Source: CAD feature listing. Evaluate the final solid. Frame: model axes, mm. Round coordinates to 2 decimals unless told otherwise and drop trailing zeros. Loops run counter-clockwise (first coordinate to the right, second up) from the corner with the lowest first, then second, coordinate; pieces in that order, holes last.
(1) First-contact query: pin 1 Ø1.9 at (x, z) = (199, 1.5) entering from -Y. Flat tip, straight axial feed; report the tip coordinate or a pass-through.
(2) Section B-B, the plane z = 0.7. Count the separate pieces of the cut face and the enclosed holes in it, plus the area to 3 significant figures.
(3) Section A-A, the plane x = 199. Return the cut outline in (y, z).
(4) Material intervals for probe 1 along Y at (x, z) = (226, 1.05); probe 2 along Y at (x, z) = (399, 3.1), sorted ascending.
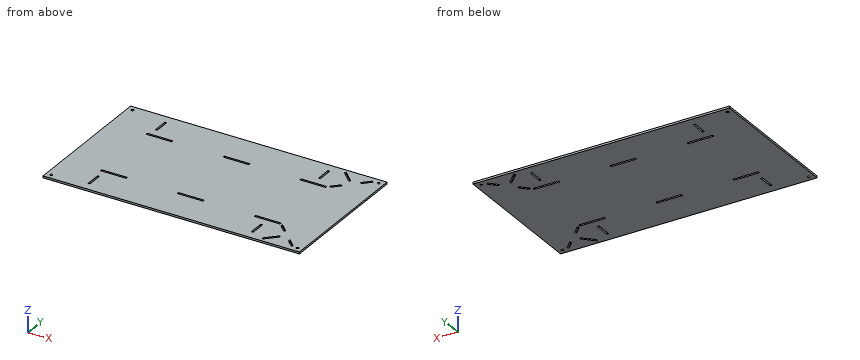
```python
from build123d import *

# Parameters (mm, degrees)
F0_W     = 3.75
F0_H     = 30
F0_W_2   = 50
F0_H_2   = 3.75
F1_DEPTH = 3.75
F3_D     = 5
F5_DEPTH = 3.75


# Not quite as in the source:
# - a feature names something its author has since deleted; it is built from what else it names


with BuildPart() as f1:
    # F0 (on Top) → F1 (new body)
    with BuildSketch(Plane.XY):
        Polygon((-37.9051826894, 0), (12.0948173106, 0), (462.0948173106, 0), (462.0948173106, 280), (62.0948173106, 280), (-37.9051826894, 280), align=None)
        with Locations((41.3065613726, 32.5)):
            Rectangle(F0_W, F0_H, mode=Mode.SUBTRACT)
        with Locations((59.4315613726, 66.875)):
            Rectangle(F0_W_2, F0_H_2, mode=Mode.SUBTRACT)
        with Locations((209.4315613726, 66.875)):
            Rectangle(F0_W_2, F0_H_2, mode=Mode.SUBTRACT)
        with Locations((359.4315613726, 32.5)):
            Rectangle(F0_W, F0_H, mode=Mode.SUBTRACT)
        with Locations((359.4315613726, 66.875)):
            Rectangle(F0_W_2, F0_H_2, mode=Mode.SUBTRACT)
        with Locations((59.4315613726, 213.125)):
            Rectangle(F0_W_2, F0_H_2, mode=Mode.SUBTRACT)
        with Locations((41.3065613726, 247.5)):
            Rectangle(F0_W, F0_H, mode=Mode.SUBTRACT)
        with Locations((209.4315613726, 213.125)):
            Rectangle(F0_W_2, F0_H_2, mode=Mode.SUBTRACT)
        with Locations((359.4315613726, 213.125)):
            Rectangle(F0_W_2, F0_H_2, mode=Mode.SUBTRACT)
        with Locations((359.4315613726, 247.5)):
            Rectangle(F0_W, F0_H, mode=Mode.SUBTRACT)
    extrude(amount=F1_DEPTH)

    # F3 (through all)
    with Locations(Plane.XY.offset(3.75)):
        with Locations((-27.9051826894, 10), (-27.9051826894, 270), (452.0948173106, 10), (452.0948173106, 270)):
            Hole(F3_D / 2)

    # F4 (on face) → F5 (cut)
    with BuildSketch(Plane.XY.offset(3.75)):
        Polygon((442.083211802, 267.3483495706), (439.4315613726, 270), (425.2894257488, 255.8578643763), (427.9410761783, 253.2062139468), align=None)
        Polygon((402.1092280247, 232.6776666521), (387.9670924009, 218.5355310284), (390.6187428304, 215.8838805989), (404.7608784541, 230.0260162227), align=None)
        Polygon((386.740880854, 273.8778619764), (384.0892304246, 271.2262115469), (405.3024338602, 250.0130081113), (407.9540842896, 252.6646585408), align=None)
        Polygon((387.9670924009, 61.4644689716), (402.1092280247, 47.3223333479), (404.7608784541, 49.9739837773), (390.6187428304, 64.1161194011), align=None)
        Polygon((405.3024338602, 29.9869918887), (384.0892304246, 8.7737884531), (386.740880854, 6.1221380236), (407.9540842896, 27.3353414592), align=None)
        Polygon((427.9410761783, 26.7937860532), (425.2894257488, 24.1421356237), (439.4315613726, 10), (442.083211802, 12.6516504294), align=None)
    extrude(amount=-F5_DEPTH, mode=Mode.SUBTRACT)


solid = f1.part
```
Output values:
1. pin 1: stops at y = 0
2. separate pieces: 1
2. enclosed holes: 20
2. area: 138,000 mm2
3. outline: (0, 0) - (65, 0) - (65, 3.75) - (0, 3.75) - close; (68.75, 0) - (211.25, 0) - (211.25, 3.75) - (68.75, 3.75) - close; (215, 0) - (280, 0) - (280, 3.75) - (215, 3.75) - close
4. probe 1: y = 0 to 65, 68.75 to 211.25, 215 to 280
4. probe 2: y = 0 to 18.38, 23.68 to 50.43, 55.73 to 224.27, 229.57 to 256.32, 261.62 to 280
